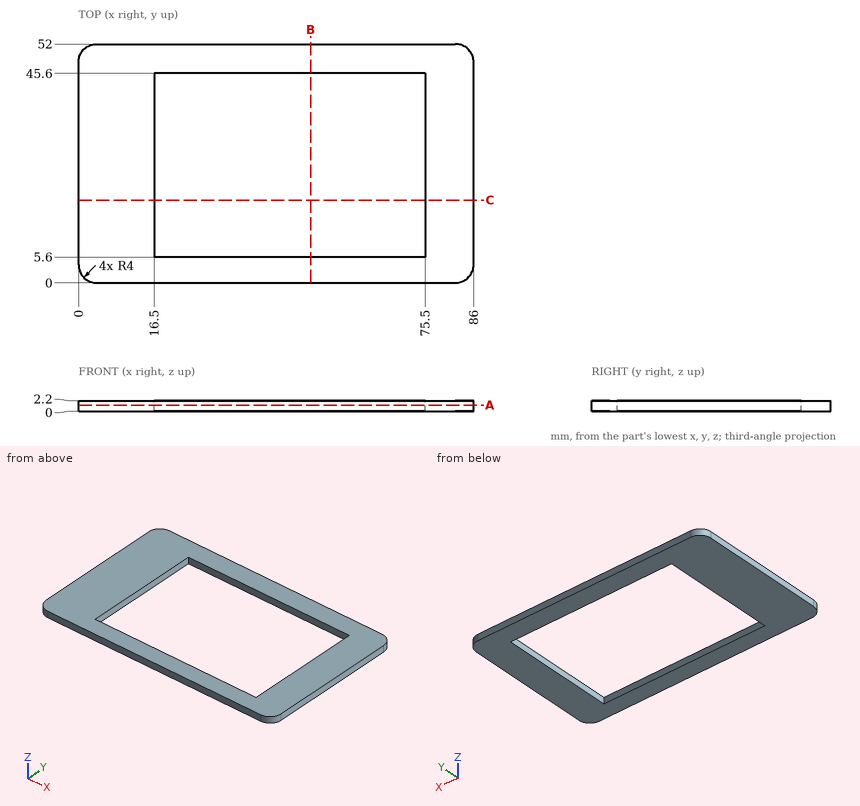
Could you check a few things on this drawing? It's one solid part, dimensions in mm from its lowest x, y, z. Give positions to 0.01 mm unless a question says otherwise; leave off trailing zeros. Order: outer loops, then holes, each group sorted by start corner. A loop starts at its lowest first (then second) coordinate and runs counter-clockwise, first axis right, second up. Notation, with made-up numbers: (-23.75, 84.25) -> (5.25, 84.25) arc R14 ccw to (5.25, 93.25) -> close; hole circle Ø7 at (57.25, 54.5). An arc over 180 degrees is marked (long way). Use CSV: the item, a comma, the result in double quotes. Start each with the question number.
Item 1: Suppose I cut it at C-C (y = 18). List the corners of the cut face in (x, z) for me, and give its area (3 significant figures).
Item 2: Suppose I cut it at B-B (x = 50.5). List the corners of the cut face in (y, z) for me, and give its area (3 significant figures).
Item 3: Suppose I cut it at A-A (z = 1.3). List the corners of the cut face in (x, y) for me, and give its area (3 significant figures).
Item 4: If I drill on probe 1 along Y at (x, z) = (51, 0.1); probe 2 along X at (y, z) = (26, 1.3), over which ranges is the centre line in solid material (lowest first)? Write a range as [from, to].
Item 5: I'm going to push a flat-ended pin straight in: P1, Ø2, axis at x = 75.5, y = 6.5, coming from the -Z side. Where does the tip first touch, or does it pass through?
Answer block:
1,outline,"(0, 0) -> (16.5, 0) -> (16.5, 2.2) -> (0, 2.2) -> close; (75.5, 0) -> (86, 0) -> (86, 2.2) -> (75.5, 2.2) -> close"
1,area,"59.4 mm^2"
2,outline,"(0, 0) -> (5.6, 0) -> (5.6, 2.2) -> (0, 2.2) -> close; (45.6, 0) -> (52, 0) -> (52, 2.2) -> (45.6, 2.2) -> close"
2,area,"26.4 mm^2"
3,outline,"(0, 4) arc R4 ccw to (4, 0) -> (82, 0) arc R4 ccw to (86, 4) -> (86, 48) arc R4 ccw to (82, 52) -> (4, 52) arc R4 ccw to (0, 48) -> close; hole (16.5, 5.6) -> (75.5, 5.6) -> (75.5, 45.6) -> (16.5, 45.6) -> close"
3,area,"2,100 mm^2"
4,probe 1,"y = [0, 5.6], [45.6, 52]"
4,probe 2,"x = [0, 16.5], [75.5, 86]"
5,P1,"stops at z = 0"
